from build123d import *

# Parameters (mm, degrees)
SKETCH_1_R      = 3
SKETCH_1_R_2    = 0.8
EXTRUDE_1_DEPTH = 2
SKETCH_2_R      = 4.5
SKETCH_2_R_2    = 3
EXTRUDE_2_DEPTH = 3


with BuildPart() as part:
    # 草圖1 → 伸長1 (new body)
    with BuildSketch(Plane(origin=(0, 0, 0), x_dir=(1, 0, 0), z_dir=(0, 1, 0))):
        with BuildLine():
            Line((0.363932704, 4.485259523), (21.75, 2.75))
            ThreePointArc((21.75, 2.75), (24.5, 0), (21.75, -2.75))
            Line((21.75, -2.75), (0.363932704, -4.485259523))
            ThreePointArc((0.363932704, -4.485259523), (-4.5, 0), (0.363932704, 4.485259523))
        make_face()
        Circle(SKETCH_1_R, mode=Mode.SUBTRACT)
        with Locations((12.75, 0)):
            Circle(SKETCH_1_R_2, mode=Mode.SUBTRACT)
        with Locations((15.75, 0)):
            Circle(SKETCH_1_R_2, mode=Mode.SUBTRACT)
        with Locations((18.75, 0)):
            Circle(SKETCH_1_R_2, mode=Mode.SUBTRACT)
        with Locations((21.75, 0)):
            Circle(SKETCH_1_R_2, mode=Mode.SUBTRACT)
    extrude(amount=EXTRUDE_1_DEPTH)

    # 草圖2 → 伸長2 (add)
    with BuildSketch(Plane.XZ.offset(-2)):
        Circle(SKETCH_2_R)
        Circle(SKETCH_2_R_2, mode=Mode.SUBTRACT)
    extrude(amount=-EXTRUDE_2_DEPTH)


solid = part.part
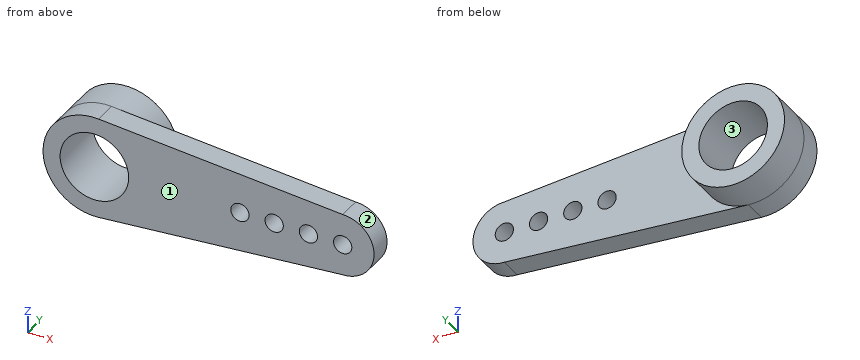
Geometry check sheet. Reference: the model listing, model coordinates, mm. Face numbers are marked on the shaded views. Round coordinates to 2 decimals unless told otherwise and drop trailing zeros. Order: outer loops, then holes, each group sorted by start corner. A loop starts at its lowest first (then second) coordinate and runs counter-clockwise, first axis right, second up. Notation, with made-up numbers: M 39,49.25 L 87,49.25 A22 cw 87,56.25 Z; hole C 13,48.25 d7. An arc over 180 degrees is marked long. Answer in a Markdown table with one row per item. Add a question column.
Item 1: Sectioned sample at C-C, the plane z = 2. Enter the section's corners in (x, y).
Item 2: Sectioned sample at B-B, the plane x = 0. Enter the section's corners in (y, z).
Item 3: Depth check by flat-ended pin: pin 1 Ø2 at (y, z) = (1, 2) entering from -X. Enter the tip coordinate at first touch or a pass-through.
Item 4: Sectioned sample at A-A, the plane z = 0. Enter the section's corners in (x, y).
Item 5: Material ranges on L1, parallel to X at y = 1.1, z = 0; L2, parallel to Z at x = 18.75, y = 1.55; L3, parallel to Z at x = 0, y = 1.45, recorded low to high. Write a range as [from, to].
Item 6: Draft check along X on the marked faces 1, 2 and 3. Enter one of: released by +X, released by -X, zero draft, split by the parting line, or undercut.
Item 7: Sectioned sample at D-D, the plane y = 2.9. Enter the section's corners in (x, z), plus the area to 3 significant figures.
Filled in:
| question | item | result |
|---|---|---|
| 1 | outline | M -4.03,0 L -2.24,0 L -2.24,5 L -4.03,5 Z; M 2.24,0 L 23.64,0 L 23.64,2 L 4.03,2 L 4.03,5 L 2.24,5 Z |
| 2 | outline | M 0,-4.5 L 5,-4.5 L 5,-3 L 0,-3 Z; M 0,3 L 5,3 L 5,4.5 L 0,4.5 Z |
| 3 | pin 1 | stops at x = -4.39 |
| 4 | outline | M -4.5,0 L -3,0 L -3,5 L -4.5,5 Z; M 3,0 L 11.95,0 L 11.95,2 L 4.5,2 L 4.5,5 L 3,5 Z; M 13.55,0 L 14.95,0 L 14.95,2 L 13.55,2 Z; M 16.55,0 L 17.95,0 L 17.95,2 L 16.55,2 Z; M 19.55,0 L 20.95,0 L 20.95,2 L 19.55,2 Z; M 22.55,0 L 24.5,0 L 24.5,2 L 22.55,2 Z |
| 5 | L1 | x = [-4.5, -3], [3, 11.95], [13.55, 14.95], [16.55, 17.95], [19.55, 20.95], [22.55, 24.5] |
| 5 | L2 | z = [-2.99, -0.8], [0.8, 2.99] |
| 5 | L3 | z = [-4.5, -3], [3, 4.5] |
| 6 | face 1 | zero draft |
| 6 | face 2 | released by +X |
| 6 | face 3 | undercut |
| 7 | outline | C 0,0 d9; hole C 0,0 d6 |
| 7 | area | 35.3 mm² |
